Print and shaded views of the part. All mm, measured from the part's lowest x, y and z. Round coordinates to 2 decimals unless told otherwise and drop trailing zeros. Loops run counter-clockwise (first coordinate to the right, second up) from the corner with the lowest first, then second, coordinate; pieces in that order, holes last. Notation, with made-up numbers: (71, 86.25) -> (100, 86.25) arc R19 cw to (100, 101.25) -> close; hole circle Ø9 at (15, 25). An arc over 180 degrees is marked (long way). Use a Markdown table: item, result.
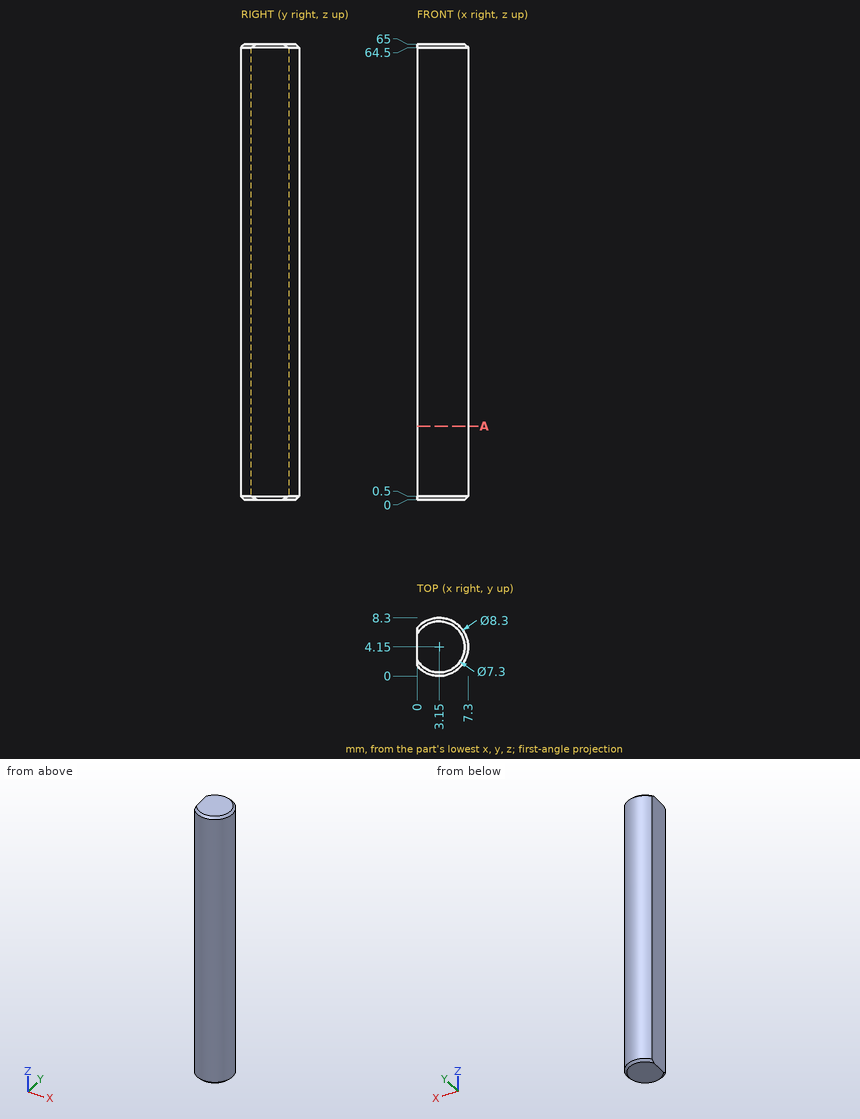
Q1. Band-saw the part on A-A, the plane z = 10.5. Give the cut face in (x, y).
Results list:
| item | result |
|---|---|
| outline | (0, 1.45) arc R4.15 ccw (long way) to (0, 6.85) -> close |
Q2. Drill centre lines: L1, parallel to Y at x = 1, z = 20.5; L2, parallel to Y at x = 5.75, z = 10.5; L3, parallel to X at y = 6.75, z = 43.5. Where is each one in solid material? Low to high. Write a range as from..to.
Results list:
| item | result |
|---|---|
| L1 | y = 0.6..7.7 |
| L2 | y = 0.92..7.38 |
| L3 | x = 0..6.38 |
Q3. Flat gauge pins, fed straight in: pin 1 (4 mm diameter, centred on x = 1, z = 38.5, fed in from -Y); pin 2 (4 mm diameter, centred on y = 1.5, z = 27, fed in from +X). Where does each tip first touch, or does it go through?
Results list:
| item | result |
|---|---|
| pin 1 | stops at y = 0 |
| pin 2 | stops at x = 7.25 |
